from build123d import *

# Parameters (mm, degrees)
SKETCH1_W           = 32.4866
SKETCH1_H           = 11.9634
SKETCH1_R           = 1.016
BOSS_EXTRUDE1_DEPTH = 2.54
SKETCH1_3_R         = 5.715
BOSS_EXTRUDE2_DEPTH = 13.4874
SKETCH2_R           = 18.034
BOSS_EXTRUDE3_DEPTH = 1.6891
SKETCH3_R           = 19.05
SKETCH3_R_2         = 0.475
CUT_EXTRUDE3_DEPTH  = 1.6891


with BuildPart() as part:
    # Sketch1 → Boss-Extrude1 (new body)
    with BuildSketch(Plane.XY):
        with Locations((-16.2433, 0)):
            Rectangle(SKETCH1_W, SKETCH1_H)
        with Locations((-2.41935, 0)):
            Circle(SKETCH1_R, mode=Mode.SUBTRACT)
        with Locations((-30.06725, 0)):
            Circle(SKETCH1_R, mode=Mode.SUBTRACT)
    extrude(amount=BOSS_EXTRUDE1_DEPTH)

    # Sketch1<3> → Boss-Extrude2 (add)
    with BuildSketch(Plane.XY):
        with Locations((-10.6045, 0)):
            Circle(SKETCH1_3_R)
    extrude(amount=-BOSS_EXTRUDE2_DEPTH)

    # Sketch2 → Boss-Extrude3 (add)
    with BuildSketch(Plane(origin=(0, 0, -13.4874), x_dir=(-1, 0, 0), z_dir=(0, 0, -1))):
        with Locations((10.6045, 0)):
            Circle(SKETCH2_R)
    extrude(amount=BOSS_EXTRUDE3_DEPTH)

    # Sketch3 → Cut-Extrude3 (cut)
    # profile 1 of 18: a face of its own
    with BuildSketch(Plane(origin=(0, 0, -15.1765), x_dir=(-1, 0, 0), z_dir=(0, 0, -1))):
        with Locations((10.6045, 0)):
            Circle(SKETCH3_R)
        with BuildLine():
            ThreePointArc((-6.2905, -1.139), (-7.4295, 0), (-6.2905, 1.139))
            Line((-6.2905, 1.139), (6.946568436, 2.752147304))
            Line((6.946568436, 2.752147304), (9.4655, 6.7095))
            ThreePointArc((9.4655, 6.7095), (10.6045, 7.8485), (11.7435, 6.7095))
            Line((11.7435, 6.7095), (14.262431564, 2.752147304))
            Line((14.262431564, 2.752147304), (25.466757758, 1.138999758))
            ThreePointArc((25.466757758, 1.138999758), (26.6065, 0), (25.466757758, -1.138999758))
            Line((25.466757758, -1.138999758), (14.262431564, -2.752147304))
            Line((14.262431564, -2.752147304), (11.7435, -6.7095))
            ThreePointArc((11.7435, -6.7095), (10.6045, -7.8485), (9.4655, -6.7095))
            Line((9.4655, -6.7095), (6.946568436, -2.752147304))
            Line((6.946568436, -2.752147304), (-6.2905, -1.139))
        make_face(mode=Mode.SUBTRACT)
    # profile 2 of 18: a face of its own
    with BuildSketch(Plane(origin=(0, 0, -15.1765), x_dir=(-1, 0, 0), z_dir=(0, 0, -1))):
        with Locations((15.3595, 0)):
            Circle(SKETCH3_R_2)
    # profile 3 of 18: a face of its own
    with BuildSketch(Plane(origin=(0, 0, -15.1765), x_dir=(-1, 0, 0), z_dir=(0, 0, -1))):
        with Locations((5.8495, 0)):
            Circle(SKETCH3_R_2)
    # profile 4 of 18: a face of its own
    with BuildSketch(Plane(origin=(0, 0, -15.1765), x_dir=(-1, 0, 0), z_dir=(0, 0, -1))):
        with Locations((17.3395, 0)):
            Circle(SKETCH3_R_2)
    # profile 5 of 18: a face of its own
    with BuildSketch(Plane(origin=(0, 0, -15.1765), x_dir=(-1, 0, 0), z_dir=(0, 0, -1))):
        with Locations((3.8695, 0)):
            Circle(SKETCH3_R_2)
    # profile 6 of 18: a face of its own
    with BuildSketch(Plane(origin=(0, 0, -15.1765), x_dir=(-1, 0, 0), z_dir=(0, 0, -1))):
        with Locations((1.8375, 0)):
            Circle(SKETCH3_R_2)
    # profile 7 of 18: a face of its own
    with BuildSketch(Plane(origin=(0, 0, -15.1765), x_dir=(-1, 0, 0), z_dir=(0, 0, -1))):
        with Locations((-0.1945, 0)):
            Circle(SKETCH3_R_2)
    # profile 8 of 18: a face of its own
    with BuildSketch(Plane(origin=(0, 0, -15.1765), x_dir=(-1, 0, 0), z_dir=(0, 0, -1))):
        with Locations((-2.2265, 0)):
            Circle(SKETCH3_R_2)
    # profile 9 of 18: a face of its own
    with BuildSketch(Plane(origin=(0, 0, -15.1765), x_dir=(-1, 0, 0), z_dir=(0, 0, -1))):
        with Locations((-4.2585, 0)):
            Circle(SKETCH3_R_2)
    # profile 10 of 18: a face of its own
    with BuildSketch(Plane(origin=(0, 0, -15.1765), x_dir=(-1, 0, 0), z_dir=(0, 0, -1))):
        with Locations((-6.2905, 0)):
            Circle(SKETCH3_R_2)
    # profile 11 of 18: a face of its own
    with BuildSketch(Plane(origin=(0, 0, -15.1765), x_dir=(-1, 0, 0), z_dir=(0, 0, -1))):
        with Locations((19.3715, 0)):
            Circle(SKETCH3_R_2)
    # profile 12 of 18: a face of its own
    with BuildSketch(Plane(origin=(0, 0, -15.1765), x_dir=(-1, 0, 0), z_dir=(0, 0, -1))):
        with Locations((21.4035, 0)):
            Circle(SKETCH3_R_2)
    # profile 13 of 18: a face of its own
    with BuildSketch(Plane(origin=(0, 0, -15.1765), x_dir=(-1, 0, 0), z_dir=(0, 0, -1))):
        with Locations((23.4355, 0)):
            Circle(SKETCH3_R_2)
    # profile 14 of 18: a face of its own
    with BuildSketch(Plane(origin=(0, 0, -15.1765), x_dir=(-1, 0, 0), z_dir=(0, 0, -1))):
        with Locations((25.4675, 0)):
            Circle(SKETCH3_R_2)
    # profile 15 of 18: a face of its own
    with BuildSketch(Plane(origin=(0, 0, -15.1765), x_dir=(-1, 0, 0), z_dir=(0, 0, -1))):
        with Locations((10.6045, 4.7295)):
            Circle(SKETCH3_R_2)
    # profile 16 of 18: a face of its own
    with BuildSketch(Plane(origin=(0, 0, -15.1765), x_dir=(-1, 0, 0), z_dir=(0, 0, -1))):
        with Locations((10.6045, -4.7295)):
            Circle(SKETCH3_R_2)
    # profile 17 of 18: a face of its own
    with BuildSketch(Plane(origin=(0, 0, -15.1765), x_dir=(-1, 0, 0), z_dir=(0, 0, -1))):
        with Locations((10.6045, 6.7095)):
            Circle(SKETCH3_R_2)
    # profile 18 of 18: a face of its own
    with BuildSketch(Plane(origin=(0, 0, -15.1765), x_dir=(-1, 0, 0), z_dir=(0, 0, -1))):
        with Locations((10.6045, -6.7095)):
            Circle(SKETCH3_R_2)
    extrude(amount=-CUT_EXTRUDE3_DEPTH, mode=Mode.SUBTRACT)


solid = part.part
Geometry: final body of the model. Coordinates: model frame, mm. A direction names the side the tool comes from. Round coordinates to 2 decimals unless told otherwise and drop trailing zeros. Loops run counter-clockwise (first coordinate to the right, second up) from the corner with the lowest first, then second, coordinate; pieces in that order, holes last. Notation, with made-up numbers: (-18.5, 57.25) - (7.5, 57.25) arc R27 ccw to (7.5, 90.25) - close; hole circle Ø8 at (72, 20.5). An arc over 180 degrees is marked (long way). Write each question's results on one line, items separated by ' | '. Start each with the question number.
1) First-contact query: P1, Ø1, axis at x = -10.5, y = 5, coming from the -Z side; P2, Ø0.8, axis at x = -7, y = 4.5, coming from the -Z side; P3, Ø1.5, axis at y = -3, z = -7.5, coming from the -X side; P4, Ø5, axis at x = -27, y = -3.5, coming from the -Z side. Flat tips, straight axial feed; report the tip coordinate or a pass-through.
2) Cut plane B-B on x = -20.5. Return loops of the section in (y, z), then the cut area to 3 significant figures.
3) Mould query, pull axis X, two halves, no side actions, for faces 6 (the face through (-6, 0, -13.487)), 7 (the face through (-4.323, 0.143, -14.344)), 8 (the face through (-8.224, -4.759, -14.344)), 9 (the face through (-10, 1, -15.176)). Classes: released by +X, released by -X, zero draft, split by the parting line, or undercut.
4) Access query for faces 1 (the face through (-0.421, -1.957, -14.344)), 2 (the face through (0, 0, 1)), 3 (the face through (-14, 4, -13.487)), 4 (the face through (-25.92, 0.14, -14.34)), 5 (the face through (-8.188, 4.703, -14.344)). Directions: +Z, -Z, +X, -X, +Y, -Y. A direction counts if a zero-diameter tool reaches every point of the face in a straight line with its end or side. Return the directions, or none.
5) Cut plane A-A on y = 0. Count the separate pieces of the cut face and the enclosed holes in it, then the cut area to 3 significant figures.
6) Cut plane C-C on y = 3.25. Return loops of the section in (x, z), then the cut area to 3 significant figures.
7) Cut plane D-D on x = -13. Return loops of the section in (y, z), then the cut area to 3 significant figures.
8) Line query: probe 1 along Z at (x, y) = (-25, 4); probe 2 along Y at (x, z) = (4, -14); probe 3 along Z at (x, y) = (-14.5, 3.75). Output: solid intervals per line, ascending. Write a range as [from, to].
Verdict:
1) P1: stops at z = -15.18 | P2: stops at z = -13.49 | P3: stops at x = -15.86 | P4: stops at z = 0
2) outline: (-5.98, 0) - (5.98, 0) - (5.98, 2.54) - (-5.98, 2.54) - close; (-1.85, -15.18) - (1.85, -15.18) - (1.85, -13.49) - (-1.85, -13.49) - close | area: 36.7 mm2
3) face 6: undercut | face 7: undercut | face 8: released by +X | face 9: zero draft
4) face 1: -Z, +X, -Y | face 2: +Z, +X, +Y, -Y | face 3: -Z, -X, +Y | face 4: -Z | face 5: -Z, +X, +Y
5) separate pieces: 14 | enclosed holes: 0 | area: 263 mm2
6) outline: (-32.49, 0) - (-15.31, 0) - (-15.31, -13.49) - (-13.95, -13.49) - (-13.95, -15.18) - (-7.26, -15.18) - (-7.26, -13.49) - (-5.9, -13.49) - (-5.9, 0) - (0, 0) - (0, 2.54) - (-32.49, 2.54) - close | area: 221 mm2
7) outline: (-5.98, 0) - (-5.19, 0) - (-5.19, -13.49) - (-4.74, -13.49) - (-4.74, -15.18) - (4.74, -15.18) - (4.74, -13.49) - (5.19, -13.49) - (5.19, 0) - (5.98, 0) - (5.98, 2.54) - (-5.98, 2.54) - close | area: 186 mm2
8) probe 1: z = [0, 2.54] | probe 2: y = [-1.42, -0.4], [0.4, 1.42] | probe 3: z = [-13.49, 2.54]
